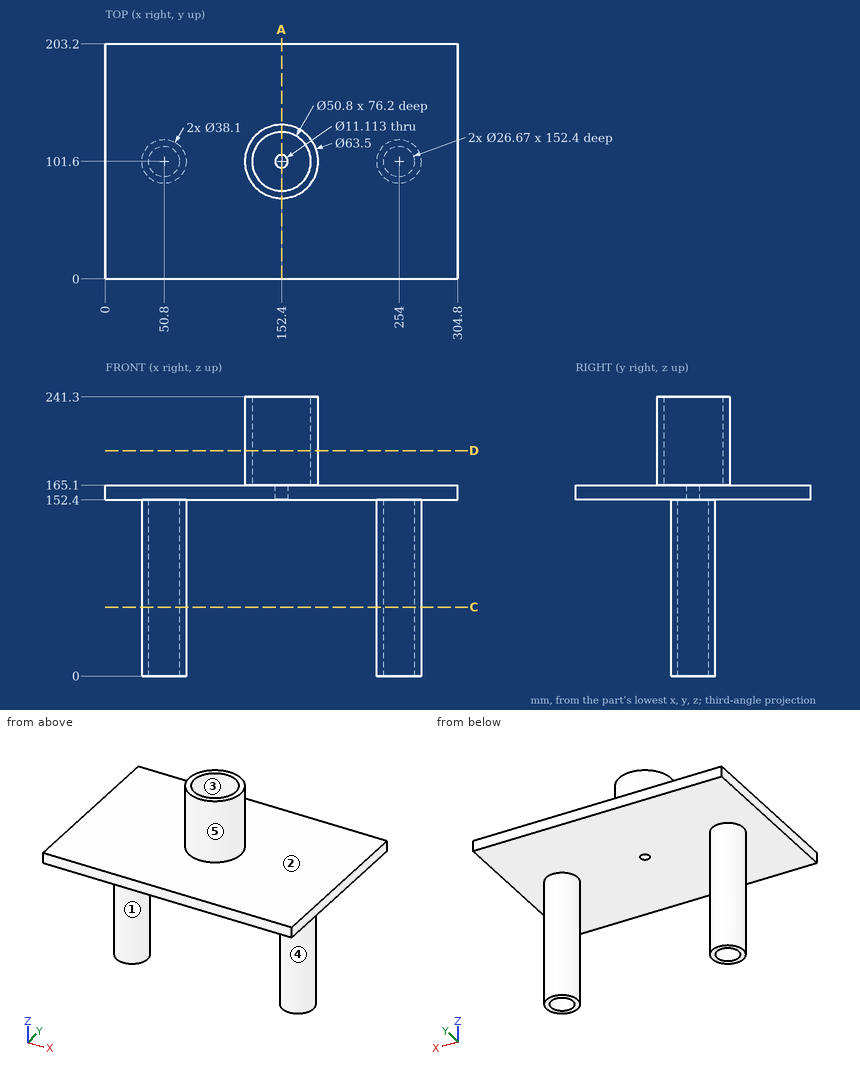
Answer from the drawing. Dimensions are ordinates in mm from the lowest x, y and z of the part. A direction names the side the tool comes from. Round coordinates to 2 decimals unless told otherwise and drop trailing zeros. Write each loop counter-clockwise with the first axis right and the second up, starting at its lowest first coordinate (ties: lowest second). Pieces come first, ordered by that corner, then holes.
1. Straight lines are drawn through the part: L1, parallel to X at y = 101, z = 76; L2, parallel to Y at x = 152.4, z = 161.75; L3, parallel to Z at x = 242, y = 105. For each, find the intervals that lie inside material, in ascending order.
2. Given pin 1 Ø1.5 at (y, z) = (122.5, 25.5) entering from -X; pin 2 Ø1.5 at (y, z) = (77, 203) entering from -X; pin 3 Ø1.5 at (x, y) = (163.5, 34) entering from +Z; pin 4 Ø8 at (x, y) = (252.5, 107) entering from -Z, each flat-ended and moving along its own axis, determine where each tip first touches the part or whether it passes through.
3. Determine the mould class of the marked faces 1, 2 and 3 for opening direction Y: pulls with the +Y half, pulls with the -Y half, needs draft (parallel to the pull), parting line crosses it, or undercut.
4. Which of the six approach directions +Z, -Z, +X, -X, +Y, -Y give full straight-line access (tool end or side, diameter ignored) to the marked faces 4 and 5?
5. The part is cut by section D-D, the plane z = 195. Determine the outline of the cut face in (x, y).
6. The part is cut by section C-C, the plane z = 59.5. State how many separate pieces and enclosed holes the cut face has, then the cut area to 3 significant figures.
7. The part is cut by section A-A, the plane x = 152.4. Determine the outline of the cut face in (y, z), then the cut area to 3 significant figures.
Values:
1. L1: x = 31.76 to 37.48, 64.12 to 69.84, 234.96 to 240.68, 267.32 to 273.04
1. L2: y = 0 to 96.04, 107.16 to 203.2
1. L3: z = 152.4 to 165.1
2. pin 1: passes through
2. pin 2: stops at x = 131.44
2. pin 3: stops at z = 165.1
2. pin 4: stops at z = 152.4
3. face 1: parting line crosses it
3. face 2: needs draft
3. face 3: undercut
4. face 4: -Z
4. face 5: +Z
5. outline: circle Ø63.5 at (152.4, 101.6); hole circle Ø50.8 at (152.4, 101.6)
6. separate pieces: 2
6. enclosed holes: 2
6. area: 1,160 mm2
7. outline: (0, 152.4) - (96.04, 152.4) - (96.04, 165.1) - (76.2, 165.1) - (76.2, 241.3) - (69.85, 241.3) - (69.85, 165.1) - (0, 165.1) - close; (107.16, 152.4) - (203.2, 152.4) - (203.2, 165.1) - (133.35, 165.1) - (133.35, 241.3) - (127, 241.3) - (127, 165.1) - (107.16, 165.1) - close
7. area: 3,410 mm2
